Could you check a few things on this model? Use its own coordinates, in mm. Face numbers are marked on the shaded views. A direction names the side the tool comes from. Give positions to 0.01 mm unless a question says otherwise; leave off trailing zeros. Write each loop counter-clockwise with the first axis right and the second up, starting at its lowest first coordinate (ties: lowest second). Pieces come first, ordered by that corner, then holes. Notation, with made-up numbers: (-3, 54) - (33, 54) arc R15 ccw to (33, 60) - close; hole circle Ø5 at (-33.75, 54.25). An arc over 180 degrees is marked (long way). Answer as CSV lines item,"result". Start each with the question number.
Q1. On a 3-axis mill with a long thin cutter (end or side, diameter ignored), from which of +Z, -Z, +X, -X, +Y, -Y can I reach the whole of each face in a straight line? I mean the marked faces 4 and 5. Say none if no direction works.
Q2. Imagine slicing it at C-C on y = 52.5. List the corners of the cut face in (x, z) for me.
Q3. Imagine slicing it at B-B on x = -0.5. List the corners of the cut face in (y, z) for me.
Q4. Will these pins go through, and if not, where does the flat tip stop? pin 1 Ø3 at (y, z) = (33, 6) entering from -X; pin 2 Ø3 at (x, z) = (24, 3.5) entering from +Y; pin 3 Ø8 at (x, y) = (27, 29) entering from +Z.
Q5. If I drill on line 1 along Y through (x, z) = (26.5, 3.5); line 2 along Z through (x, y) = (18, 15); line 3 along Y through (x, z) = (2.5, 4.75), over which ranges is the centre line in solid material (lowest first)?
Q6. We'd pull the mould along X, two halves only. Please class the marked faces 1, 2 and 3: pulls with the +X half, pulls with the -X half, needs draft (parallel to the pull), parting line crosses it, or undercut.
Q7. Imagine slicing it at A-A on z = 5.5. List the corners of the cut face in (x, y) for me.
```python
from build123d import *

# Parameters (mm, degrees)
BOSS_EXTRUDE2_DEPTH = 1.5875
BOSS_EXTRUDE3_DEPTH = 7.9375


with BuildPart() as part:
    # Sketch1 → Boss-Extrude2 (new body)
    with BuildSketch(Plane.XY):
        Polygon((33.217447351, 54.34868871), (33.217447351, 13.07368871), (-13.137552649, 13.07368871), align=None)
    extrude(amount=BOSS_EXTRUDE2_DEPTH)

    # Sketch1<5> → Boss-Extrude3 (add)
    with BuildSketch(Plane.XY):
        Polygon((34.487447351, 57.364746686), (34.487447351, 11.80368871), (-16.171808963, 11.80368871), align=None)
        Polygon((33.217447351, 54.34868871), (33.217447351, 13.07368871), (-13.137552649, 13.07368871), align=None, mode=Mode.SUBTRACT)
    extrude(amount=BOSS_EXTRUDE3_DEPTH)


solid = part.part
```
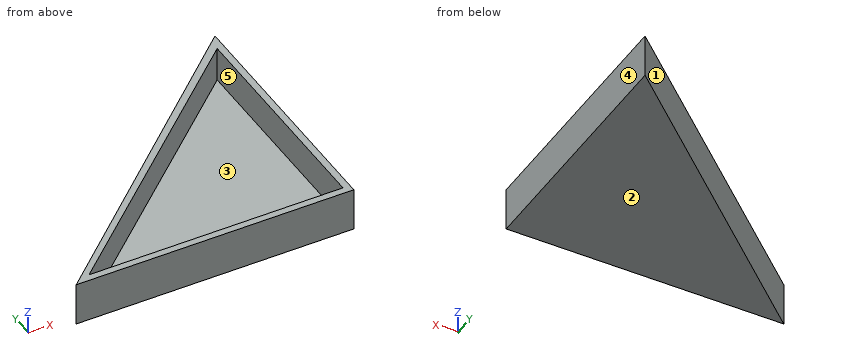
Conclusion:
1,face 4,"+Z, -Z, +X, +Y, -Y"
1,face 5,"+Z"
2,outline,"(29.08, 0) - (34.49, 0) - (34.49, 7.94) - (33.22, 7.94) - (33.22, 1.59) - (31.14, 1.59) - (31.14, 7.94) - (29.08, 7.94) - close"
3,outline,"(11.8, 0) - (25.9, 0) - (25.9, 7.94) - (24.33, 7.94) - (24.33, 1.59) - (13.07, 1.59) - (13.07, 7.94) - (11.8, 7.94) - close"
4,pin 1,"x = 5.73"
4,pin 2,"y = 49.28"
4,pin 3,"z = 1.59"
5,line 1,"11.8 to 13.07, 48.37 to 50.18"
5,line 2,"0 to 1.59"
5,line 3,"11.8 to 13.07, 27 to 28.6"
6,face 1,"pulls with the -X half"
6,face 2,"needs draft"
6,face 3,"undercut"
7,outline,"(-16.17, 11.8) - (34.49, 11.8) - (34.49, 57.36) - close; hole (-13.14, 13.07) - (33.22, 13.07) - (33.22, 54.35) - close"
